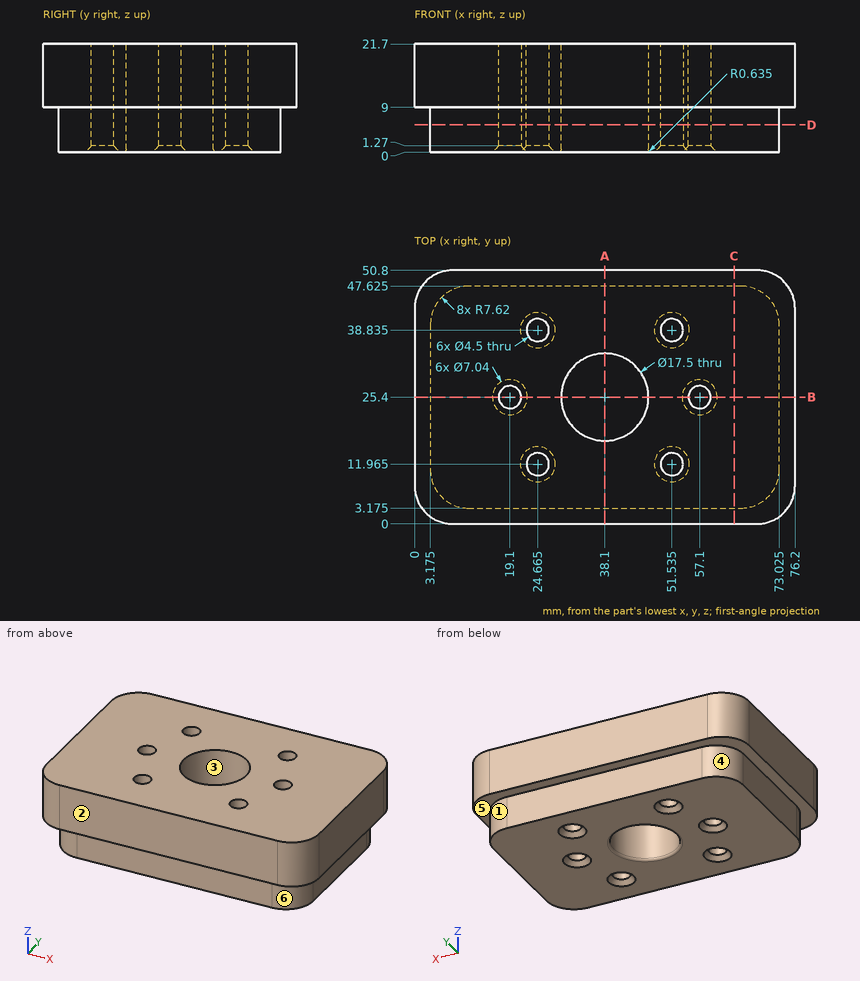
Source: three-view drawing plus pictorial views. Frame: mm from the lowest corner of the part. A direction names the side the tool comes from. Coordinates: 2 decimals unless noted, no trailing zeros. Loops run counter-clockwise (first coordinate to the right, second up) from the corner with the lowest first, then second, coordinate; pieces in that order, holes last. Notation, with made-up numbers: (44.5, 33) -> (97.5, 33) arc R22 ccw to (97.5, 68) -> close; hole circle Ø6 at (3, -1). An arc over 180 degrees is marked (long way). Write each question's results on one line, items separated by ' | '. Start each with the question number.
Q1. Reachability of the marked faces 4, 5 and 6 from +Z, -Z, +X, -X, +Y, -Y: full face, straight path, thin tool, end or side. Return the list, or none.
Q2. Section A-A, the plane x = 38.1. Return the cut outline in (y, z) (3 decimals), plus the area to 3 significant figures.
Q3. Section B-B, the plane y = 25.4. Return the cut outline in (x, z) (3 decimals), plus the area to 3 significant figures.
Q4. Ray query, line 1 (Y direction, x = 49.5, z = 11.5); line 2 (X direction, y = 14, z = 5.25) (3 decimals); line 3 (X direction, y = 23.5, z = 1) (3 decimals). Return the intervals inside material, ascending. Write a range as from..to.
Q5. Section D-D, the plane z = 5.5. Return the cut outline in (x, y) (3 decimals).
Q6. Section C-C, the plane x = 64. Return the cut outline in (y, z) (3 decimals), plus the area to 3 significant figures.
Q7. Pull-direction query (Y, two-part tool) for the marked faces 1, 2 and 3; classes: released by +Y, released by -Y, zero draft, split by the parting line, or undercut.
Q8. Pin query (flat end, axial travel): pin 1 (3 mm diameter, centred on x = 11, z = 14, fed in from -Y); pin 2 (4.5 mm diameter, centred on x = 28.5, z = 5.5, fed in from +Y) (3 decimals); pin 3 (7 mm diameter, centred on x = 36.5, z = 4.5, fed in from -Y) (3 decimals); pin 4 (2.5 mm diameter, centred on y = 21, z = 6, fed in from +X) (3 decimals). Return the tip coordinate at first contact, or that it passes through.
Found:
1) face 4: -Z, -X, +Y | face 5: -Z | face 6: -Z, +X, -Y
2) outline: (0, 9) -> (3.175, 9) -> (3.175, 0) -> (16.015, 0) arc R0.635 ccw to (16.65, 0.635) -> (16.65, 21.7) -> (0, 21.7) -> close; (34.15, 0.635) arc R0.635 ccw to (34.785, 0) -> (47.625, 0) -> (47.625, 9) -> (50.8, 9) -> (50.8, 21.7) -> (34.15, 21.7) -> close | area: 665 mm2
3) outline: (0, 9) -> (3.175, 9) -> (3.175, 0) -> (15.58, 0) -> (16.85, 1.27) -> (16.85, 21.7) -> (0, 21.7) -> close; (21.35, 1.27) -> (22.62, 0) -> (28.715, 0) arc R0.635 ccw to (29.35, 0.635) -> (29.35, 21.7) -> (21.35, 21.7) -> close; (46.85, 0.635) arc R0.635 ccw to (47.485, 0) -> (53.58, 0) -> (54.85, 1.27) -> (54.85, 21.7) -> (46.85, 21.7) -> close; (59.35, 1.27) -> (60.62, 0) -> (73.025, 0) -> (73.025, 9) -> (76.2, 9) -> (76.2, 21.7) -> (59.35, 21.7) -> close | area: 1,020 mm2
4) line 1: 0..11.01, 12.92..37.88, 39.79..50.8 | line 2: 3.175..23.705, 25.625..50.575, 52.495..73.025 | line 3: 3.175..17.445, 20.755..29.559, 46.641..55.445, 58.755..73.025
5) outline: (3.175, 10.795) arc R7.62 ccw to (10.795, 3.175) -> (65.405, 3.175) arc R7.62 ccw to (73.025, 10.795) -> (73.025, 40.005) arc R7.62 ccw to (65.405, 47.625) -> (10.795, 47.625) arc R7.62 ccw to (3.175, 40.005) -> close; hole circle Ø4.5 at (19.1, 25.4); hole circle Ø4.5 at (24.665, 11.965); hole circle Ø4.5 at (24.665, 38.835); hole circle Ø17.5 at (38.1, 25.4); hole circle Ø4.5 at (51.535, 11.965); hole circle Ø4.5 at (51.535, 38.835); hole circle Ø4.5 at (57.1, 25.4)
6) outline: (0, 9) -> (3.175, 9) -> (3.175, 0) -> (47.625, 0) -> (47.625, 9) -> (50.8, 9) -> (50.8, 21.7) -> (0, 21.7) -> close | area: 1,050 mm2
7) face 1: released by +Y | face 2: released by -Y | face 3: undercut
8) pin 1: y = 0 | pin 2: y = 47.625 | pin 3: y = 3.175 | pin 4: x = 73.025
